```python
from build123d import *

# Parameters (mm, degrees)
BOSS_EXTRUDE1_DEPTH    = 49
FILLET1_R              = 5
CUT_EXTRUDE1_START     = -2.282608696
CUT_EXTRUDE1_OUTLINE_W = 10
CUT_EXTRUDE1_OUTLINE_H = 37
CUT_EXTRUDE1_DEPTH     = 13
SKETCH6_R              = 2
BOSS_EXTRUDE2_DEPTH    = 37
CUT_EXTRUDE2_DEPTH     = 49


# Read off the part's stored shape, not the designer's step: Cut-Extrude1
with BuildPart() as part:
    # Sketch3 → Boss-Extrude1 (new body)
    with BuildSketch(Plane.XY.offset(24.5)):
        Polygon((-5, -2.282608696), (0, -2.282608696), (5, -2.282608696), (5, 49.717391304), (-5, 49.717391304), align=None)
    extrude(amount=-BOSS_EXTRUDE1_DEPTH)

    # Fillet1
    fillet1_edges = [part.edges().sort_by_distance(p)[0] for p in [
        (5, -2.282608696, 0),
        (-5, -2.282608696, 0),
        (5, 49.717391304, 0),
        (-5, 49.717391304, 0),
    ]]
    fillet(fillet1_edges, radius=FILLET1_R - 0.0001)  # a hair under: the kernel refuses the full size

    # Cut-Extrude1 outline → Cut-Extrude1 (cut)
    with BuildSketch(Plane(origin=(0, 0, 0), x_dir=(1, 0, 0), z_dir=(0, 1, 0)).offset(CUT_EXTRUDE1_START)):
        Rectangle(CUT_EXTRUDE1_OUTLINE_W, CUT_EXTRUDE1_OUTLINE_H)
    extrude(amount=CUT_EXTRUDE1_DEPTH, mode=Mode.SUBTRACT)

    # Sketch6 → Boss-Extrude2 (add)
    with BuildSketch(Plane.XY.offset(-18.5)):
        with Locations((0, 2.717391304)):
            Circle(SKETCH6_R)
    extrude(amount=BOSS_EXTRUDE2_DEPTH)

    # Sketch7 → Cut-Extrude2 (cut)
    with BuildSketch(Plane.XY.offset(24.5)):
        with BuildLine():
            Line((4.5, 3.717391304), (5, 3.717391304))
            Line((5, 3.717391304), (5, 2.717391304))
            ThreePointArc((5, 2.717391304), (3.535533906, -0.818142602), (0, -2.282608696))
            ThreePointArc((0, -2.282608696), (-3.535533906, -0.818142602), (-5, 2.717391304))
            Line((-5, 2.717391304), (-5, 18.717391304))
            Line((-5, 18.717391304), (-4.5, 18.717391304))
            Line((-4.5, 18.717391304), (-4.5, 2.717391304))
            ThreePointArc((-4.5, 2.717391304), (-3.181980515, -0.464589211), (0, -1.782608696))
            ThreePointArc((0, -1.782608696), (3.181980515, -0.464589211), (4.5, 2.717391304))
            Line((4.5, 2.717391304), (4.5, 3.717391304))
        make_face()
    extrude(amount=-CUT_EXTRUDE2_DEPTH, mode=Mode.SUBTRACT)


with BuildPart() as cut_extrude2_kept_piece:
    # of the separate pieces the step leaves, the one the design keeps (cut_extrude2_pieces_kept)
    add(part.part.solids().sort_by_distance((4.5, 3.717391304, -18.5))[0])


solid = cut_extrude2_kept_piece.part
```
Check sheet for the modelled part. Datum: model origin and axes. Units: mm. A direction names the side the tool comes from. Give positions to 0.01 mm unless a question says otherwise; leave off trailing zeros. Order: outer loops, then holes, each group sorted by start corner. A loop starts at its lowest first (then second) coordinate and runs counter-clockwise, first axis right, second up. Notation, with made-up numbers: M 81.25,-1.5 L 103.25,-1.5 A17 cw 103.25,2.5 Z; hole C 76,-6 d5. An arc over 180 degrees is marked long. Answer in a Markdown table with one row per item. Add a question column.
Q1. Sectioned sample at B-B, the plane x = 1. Record the boundary of the cut face in (y, z), and give its area (3 significant figures).
Q2. Access from +Z, -Z, +X, -X, +Y, -Y to the whole of each face (thin tool, end or side, straight path). Record for faces 1 (the flat face through (0, 10.717, 0)), 2 (the cylindrical face through (-3.5, 48.29, -0.34)), 3 (the cylindrical face through (-0.434, 0.765, -0.259)), 4 (the flat face through (-4.5, 13, 0)).
Q3. Sectioned sample at C-C, the plane y = 16. Record the boundary of the cut face in (x, z).
Q4. Thickness scan on L1, parallel to Z at x = -2.5, y = 0; L2, parallel to Y at x = 0, z = 17.5; L3, parallel to Y at x = -1, z = 2. Record the ranges inside material, lowest first.
Q5. Sectioned sample at D-D, the plane x = -3.5. Record the boundary of the cut face in (y, z), and give its area (3 significant figures).
Q6. Gauge pin test, flat ends, axial feed: pin 1 Ø0.8 at (y, z) = (3, -21.5) entering from +X; pin 2 Ø3 at (x, z) = (1.5, -7.5) entering from -Y; pin 3 Ø6 at (x, z) = (-3.5, -11.5) entering from +Y. Record the tip position at first contact, or that the pin passes through.
Q7. Release check for a two-part mould opening along Z. For faces 5 (the flat face through (0, 24, 24.5)), 6 (the flat face through (0, 6, 18.5)), 7 (the flat face through (0, 24, -24.5)), 8 (the cylindrical face through (3.574, 48.214, -0.343)) record: released by +Z, released by -Z, zero draft, split by the parting line, or undercut.
Verdict:
| question | item | result |
|---|---|---|
| 1 | outline | M -1.67,-24.5 L 49.62,-24.5 L 49.62,24.5 L -1.67,24.5 L -1.67,18.5 L 0.99,18.5 L 0.99,-18.5 L -1.67,-18.5 Z; hole M 4.45,-18.5 L 10.72,-18.5 L 10.72,18.5 L 4.45,18.5 Z |
| 1 | area | 2,180 mm² |
| 2 | face 1 | +X, -X |
| 2 | face 2 | +Z, -Z, -X, +Y |
| 2 | face 3 | none |
| 2 | face 4 | +Z, -Z, -X, -Y |
| 3 | outline | M -4.5,-24.5 L 5,-24.5 L 5,24.5 L -4.5,24.5 Z |
| 4 | L1 | -24.5 to -18.5, 18.5 to 24.5 |
| 4 | L2 | 0.72 to 4.72, 10.72 to 49.72 |
| 4 | L3 | 0.99 to 4.45, 10.72 to 49.62 |
| 5 | outline | M -0.11,-24.5 L 48.29,-24.5 L 48.29,24.5 L -0.11,24.5 L -0.11,18.5 L 10.72,18.5 L 10.72,-18.5 L -0.11,-18.5 Z |
| 5 | area | 1,970 mm² |
| 6 | pin 1 | x = 4.5 |
| 6 | pin 2 | y = 0.72 |
| 6 | pin 3 | y = 49.69 |
| 7 | face 5 | released by +Z |
| 7 | face 6 | undercut |
| 7 | face 7 | released by -Z |
| 7 | face 8 | zero draft |
